For this review, use the dimensioned drawing (mm, ordinates from the lowest corner) and the shaded views. A direction names the side the tool comes from. Coordinates: 2 decimals unless noted, no trailing zeros. Write each loop counter-clockwise with the first axis right and the second up, starting at its lowest first coordinate (ties: lowest second). Pieces come first, ordered by that corner, then holes. Notation, with made-up numbers: (-28.5, -34) - (-16.5, -34) arc R9 cw to (-16.5, -23) - close; hole circle Ø7 at (3.5, 23.25). An arc over 180 degrees is marked (long way). One line per item, written item: value.
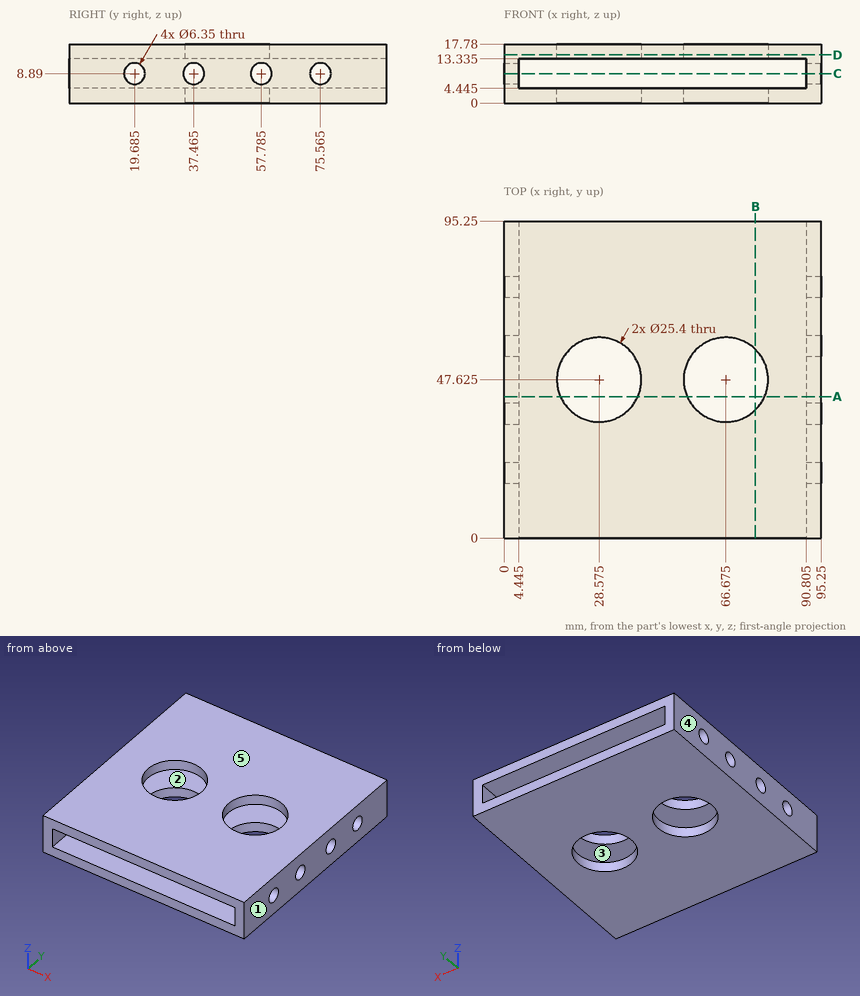
1. Wall thickness on line 1 along Y through (x, z) = (3.5, 8.89); line 2 along X through (y, z) = (24.5, 11.25) (3 decimals); line 3 along Z through (x, y) = (57.5, 73) (3 decimals): over which ranges is each line inside the solid? List them lowest first.
Answer block:
line 1: y = 0 to 16.51, 22.86 to 34.29, 40.64 to 54.61, 60.96 to 72.39, 78.74 to 95.25
line 2: x = 0 to 4.445, 90.805 to 95.25
line 3: z = 0 to 4.445, 13.335 to 17.78
2. Consider section A-A, the plane y = 42.5. Write out the cut boundary in (x, z) (3 decimals), then the cut area to 3 significant figures.
Answer block:
outline: (0, 0) - (16.955, 0) - (16.955, 4.445) - (4.445, 4.445) - (4.445, 13.335) - (16.955, 13.335) - (16.955, 17.78) - (0, 17.78) - close; (40.195, 0) - (55.055, 0) - (55.055, 4.445) - (40.195, 4.445) - close; (40.195, 13.335) - (55.055, 13.335) - (55.055, 17.78) - (40.195, 17.78) - close; (78.295, 0) - (95.25, 0) - (95.25, 17.78) - (78.295, 17.78) - (78.295, 13.335) - (90.805, 13.335) - (90.805, 4.445) - (78.295, 4.445) - close
area: 513 mm^2
3. For the marked faces 1 and 2, list the 3-axis set-ups (+Z, -Z, +X, -X, +Y, -Y) from which the entire face can be reached by the end or side of a thin tool; tool diameter is ignored.
Answer block:
face 1: +Z, -Z, +X, +Y, -Y
face 2: +Y, -Y
4. Consider section B-B, the plane x = 75.5. Write out the cut boundary in (y, z) (3 decimals), then the cut area to 3 significant figures.
Answer block:
outline: (0, 0) - (38.492, 0) - (38.492, 4.445) - (0, 4.445) - close; (0, 13.335) - (38.492, 13.335) - (38.492, 17.78) - (0, 17.78) - close; (56.758, 0) - (95.25, 0) - (95.25, 4.445) - (56.758, 4.445) - close; (56.758, 13.335) - (95.25, 13.335) - (95.25, 17.78) - (56.758, 17.78) - close
area: 684 mm^2
5. Consider section C-C, the plane z = 8.89. Give the number of separate pieces and of enclosed holes in the cut face, then the cut area to 3 significant figures.
Answer block:
separate pieces: 10
enclosed holes: 0
area: 621 mm^2
6. Consider section D-D, the plane z = 14.5. Write out the cut boundary in (x, y) (3 decimals), then the cut area to 3 significant figures.
Answer block:
outline: (0, 0) - (95.25, 0) - (95.25, 95.25) - (0, 95.25) - close; hole circle Ø25.4 at (28.575, 47.625); hole circle Ø25.4 at (66.675, 47.625)
area: 8,060 mm^2
7. Mouldability with a two-part tool opening along Z and no side actions: class the marked faces 3, 4 and 5 as released by +Z, released by -Z, zero draft, split by the parting line, or undercut.
Answer block:
face 3: undercut
face 4: zero draft
face 5: released by +Z
